Check sheet for the modelled part. Datum: model origin and axes. Units: mm. A direction names the side the tool comes from. Round coordinates to 2 decimals unless told otherwise and drop trailing zeros. Loops run counter-clockwise (first coordinate to the right, second up) from the corner with the lowest first, then second, coordinate; pieces in that order, holes last. Notation, with made-up numbers: (-14.5, 52) -> (-3.5, 52) arc R18 ccw to (-3.5, 60) -> close; hole circle Ø10 at (48, 10.5). An arc over 180 degrees is marked (long way). Return JSON: item names as keys, results as strings.
from build123d import *

# Parameters (mm, degrees)
CYLINDER053_R                     = 1.75
CYLINDER053_DEPTH                 = 15
CYLINDER052_R                     = 1.75
CYLINDER052_DEPTH                 = 15
EXTRUDE003_DEPTH                  = 10
FILLET021_R                       = 1
EXTRUDE004_DEPTH                  = 5
PART_MIRRORING006_PLACEMENT_ANGLE = 180


with BuildPart() as m3holds021:
    # Cylinder053 → Cylinder053 (new body)
    with BuildSketch(Plane(origin=(72, 0.25, -9), x_dir=(1, 0, 0), z_dir=(0, -1, 0))):
        Circle(CYLINDER053_R)
    extrude(amount=CYLINDER053_DEPTH)


with BuildPart() as fusion064:
    # Cylinder052 → Cylinder052 (new body)
    with BuildSketch(Plane(origin=(63.6, 0.25, 3.5), x_dir=(1, 0, 0), z_dir=(0, -1, 0))):
        Circle(CYLINDER052_R)
    extrude(amount=CYLINDER052_DEPTH)

    # Fusion064: union m3Holds021
    add(m3holds021.part)


with BuildPart() as fillet021:
    # Sketch005 → Extrude003 (new body)
    with BuildSketch(Plane.XY):
        Polygon((57.709053, -19.346786), (57.709053, -22.346786), (65.709053, -22.346786), (65.709053, -10.346786), (62.709053, -10.346786), (62.709053, -19.346786), align=None)
    extrude(amount=EXTRUDE003_DEPTH)


with BuildPart() as fillet021_1:
    # Extrude003 placement: moved
    add(fillet021.part.moved(Location((0, 0, -14))))

    # Fillet021
    fillet021_edges = [fillet021_1.edges().sort_by_distance(p)[0] for p in [
        (57.709053, -19.346786, -9),
        (57.709053, -22.346786, -9),
        (65.709053, -22.346786, -9),
        (61.709053, -22.346786, -4),
        (65.709053, -10.346786, -9),
        (65.709053, -16.346786, -4),
        (62.709053, -10.346786, -9),
        (64.209053, -10.346786, -4),
        (62.709053, -19.346786, -9),
        (62.709053, -14.846786, -4),
        (60.209053, -19.346786, -4),
    ]]
    fillet(fillet021_edges, radius=FILLET021_R)


with BuildPart() as fillet021_2:
    # Fillet021 placement: moved
    add(fillet021_1.part.moved(Location((0, 0, 0.4))))


with BuildPart() as extrude004:
    # Sketch006 → Extrude004 (new body)
    with BuildSketch(Plane.XZ):
        with BuildLine():
            ThreePointArc((14.771842, 0.154152), (17.827348, 3.62591), (14.461083, 6.797264))
            Line((14.461083, 6.797264), (12.252875, 6.797264))
            Line((12.252875, -5.267611), (12.252875, 6.797264))
            Line((5.422805, -5.82309), (12.252875, -5.267611))
            ThreePointArc((5.422805, -5.82309), (2.802341, -9.576998), (6.556249, -12.197462))
            Line((6.556249, -12.197462), (14.771842, -12.197462))
            Line((14.771842, -12.197462), (14.771842, 0.154152))
        make_face()
    extrude(amount=EXTRUDE004_DEPTH)


with BuildPart() as extrude004_1:
    # Extrude004 placement: moved
    add(extrude004.part.moved(Location((0, -8, 0))))


with BuildPart() as obj1:
    # Part__Mirroring006: instance of Extrude004
    add(extrude004_1.part.mirror(Plane(origin=(0, 0, 0), x_dir=(0, 1, 0), z_dir=(0, 0, 1))))


with BuildPart() as obj1_1:
    # Part__Mirroring006 placement: moved
    add(obj1.part.moved(Location((78, 0, 0))).rotate(Axis((78, 0, 0), (0, 1, 0)), PART_MIRRORING006_PLACEMENT_ANGLE))

    # Fusion041: union Fillet021
    add(fillet021_2.part)

    # Cut014: cut Fusion064
    add(fusion064.part, mode=Mode.SUBTRACT)


solid = obj1_1.part
Q1. Section check D-D (y = -14). Record the boundary of the cut face in (x, z).
Results list:
{"outline": "(62.71, -13.6) -> (65.71, -13.6) -> (65.71, -4.6) arc R1 ccw to (64.71, -3.6) -> (63.71, -3.6) arc R1 ccw to (62.71, -4.6) -> close"}
Q2. Section check C-C (z = -8.75). Record the boundary of the cut face in (x, y), then the cut area to 3 significant figures.
Results list:
{"outline": "(57.71, -21.35) arc R1 ccw to (58.71, -22.35) -> (64.71, -22.35) arc R1 ccw to (65.71, -21.35) -> (65.71, -13) -> (70.27, -13) -> (70.27, -8) -> (63.23, -8) -> (63.23, -10.47) arc R1 ccw to (62.71, -11.35) -> (62.71, -18.35) arc R1 cw to (61.71, -19.35) -> (58.71, -19.35) arc R1 ccw to (57.71, -20.35) -> close; (73.73, -13) -> (75.24, -13) -> (75.24, -8) -> (73.73, -8) -> close", "area": "86.5 mm^2"}
Q3. Draft check along X on faces 1 (the cylindrical face through (62.9, -10.76, -9.04)), 2 (the flat face through (68, -10, -12.197)), 3 (the cylindrical face through (65.424, -17.115, -3.901)), 4 (the flat face through (64, -19, -3.6)). Enter one of: released by +X, released by -X, zero draft, split by the parting line, or undercut.
Results list:
{"face 1": "released by -X", "face 2": "undercut", "face 3": "released by +X", "face 4": "zero draft"}
Q4. Section check B-B (x = 61). Record the boundary of the cut face in (y, z).
Results list:
{"outline": "(-22.35, -13.6) -> (-19.35, -13.6) -> (-19.35, -4.6) arc R1 ccw to (-20.35, -3.6) -> (-21.35, -3.6) arc R1 ccw to (-22.35, -4.6) -> close; (-13, 1.27) -> (-8, 1.27) -> (-8, 5.67) -> (-13, 5.67) -> close"}
Q5. Go/stop test with flat-tipped pins: pin 1 (2.5 mm diameter, centred on x = 61, z = -11, fed in from +Y); pin 2 (5.5 mm diameter, centred on y = -10, z = -2, fed in from +X); pin 3 (8 mm diameter, centred on x = 63, y = -9.5, fed in from -Z); pin 4 (0.8 mm diameter, centred on x = 64.5, z = -13, fed in from +Y). Record where each tip stops, or that it passes through.
Results list:
{"pin 1": "y = -19.19", "pin 2": "x = 65.75", "pin 3": "z = -13.6", "pin 4": "y = -10.35"}
Q6. Tool access check on faces 5 (the flat face through (62.709, -15, -9)), 6 (the flat face through (65.747, -10, 1)), 7 (the flat face through (60, -19.347, -9)), 8 (the cylindrical face through (59.68, -19.63, -3.9)). Record the directions out of +Z, -Z, +X, -X, +Y, -Y that give a thin tool (end or side, any length) a straight path to the whole face; none if there is none.
Results list:
{"face 5": "-Z, -X, +Y", "face 6": "+Z, +X, +Y, -Y", "face 7": "+Z, -Z, -X, +Y", "face 8": "+Z, -X, +Y"}
Q7. Section check A-A (y = -12). Record the boundary of the cut face in (x, z).
Results list:
{"outline": "(62.71, -13.6) -> (65.71, -13.6) -> (65.71, -12.2) -> (71.44, -12.2) arc R3.24 ccw to (72.58, -5.82) -> (65.75, -5.27) -> (65.75, 6.8) -> (63.54, 6.8) arc R3.33 ccw to (63.23, 0.15) -> (63.23, -3.72) arc R1 ccw to (62.71, -4.6) -> close; hole circle Ø3.5 at (63.6, 3.5); hole circle Ø3.5 at (72, -9)"}
Q8. Material ranges on line 1 (X direction, y = -10.3, z = 3.5); line 2 (X direction, y = -11.6, z = -9); line 3 (Z direction, x = 63.6, y = -9.4), recorded low to high.
Results list:
{"line 1": "60.17 to 61.85, 65.35 to 65.75", "line 2": "62.71 to 70.25, 73.75 to 75.25", "line 3": "-12.2 to 1.75, 5.25 to 6.8"}
